from build123d import *

# Parameters (mm, degrees)
SKETCH1_R           = 18
BOSS_EXTRUDE1_DEPTH = 5
SKETCH2_R           = 18
SKETCH2_R_2         = 16.7
BOSS_EXTRUDE2_DEPTH = 25
SKETCH3_W           = 4
SKETCH3_H           = 4.625561496
CUT_EXTRUDE1_DEPTH  = 25


with BuildPart() as part:
    # Sketch1 → Boss-Extrude1 (new body)
    with BuildSketch(Plane(origin=(0, 0, 0), x_dir=(1, 0, 0), z_dir=(0, 1, 0))):
        with Locations(Location((0, 0, 0), (0, 0, 270))):
            Circle(SKETCH1_R)
    extrude(amount=BOSS_EXTRUDE1_DEPTH)

    # Sketch2 → Boss-Extrude2 (add)
    with BuildSketch(Plane(origin=(0, 5, 0), x_dir=(1, 0, 0), z_dir=(0, 1, 0))):
        with Locations(Location((0, 0, 0), (0, 0, 270))):
            Circle(SKETCH2_R)
        with Locations(Location((0, 0, 0), (0, 0, 270))):
            Circle(SKETCH2_R_2, mode=Mode.SUBTRACT)
    extrude(amount=BOSS_EXTRUDE2_DEPTH)

    # Sketch3 → Cut-Extrude1 (cut)
    with BuildSketch(Plane(origin=(0, 30, 0), x_dir=(1, 0, 0), z_dir=(0, 1, 0))):
        with Locations((0, 16.7)):
            Rectangle(SKETCH3_W, SKETCH3_H)
    extrude(amount=-CUT_EXTRUDE1_DEPTH, mode=Mode.SUBTRACT)

    # Cut-Loft1: read off the stored shape, not the designer's step
    # Cut-Loft1: loft between two sections, ruled curve by curve
    cut_loft1_from = [
        Edge.make_bspline([(-1.712462043, 0, -8.966813787), (-1.626363192, 0, -8.824108617), (-1.511615223, 0, -8.673150149), (-1.197727621, 0, -8.384153579), (-0.9972614, 0, -8.245981525), (-0.502854414, 0, -8.045966083), (-0.20751606, 0, -7.986207367), (0.419056865, 0, -8.019390239), (0.747775872, 0, -8.115340255), (1.318596553, 0, -8.459735659), (1.556747911, 0, -8.705797688), (1.878250858, 0, -9.244621024), (1.963090928, 0, -9.533754229), (2.016671796, 0, -10.064389259), (1.987908436, 0, -10.306155451), (1.878602966, 0, -10.718583333), (1.798560894, 0, -10.890481042), (1.626363192, 0, -11.175891383), (1.511615223, 0, -11.326849851), (1.197727621, 0, -11.615846421), (0.9972614, 0, -11.754018475), (0.502854414, 0, -11.954033917), (0.20751606, 0, -12.013792633), (-0.419056865, 0, -11.980609761), (-0.747775872, 0, -11.884659745), (-1.318596553, 0, -11.540264341), (-1.556747911, 0, -11.294202312), (-1.878250858, 0, -10.755378976), (-1.963090928, 0, -10.466245771), (-2.016671796, 0, -9.935610741), (-1.987908436, 0, -9.693844549), (-1.878602966, 0, -9.281416667), (-1.798560894, 0, -9.109518958), (-1.712462043, 0, -8.966813787)], [0, 0, 0, 0, 0.0625, 0.0625, 0.125, 0.125, 0.1875, 0.1875, 0.25, 0.25, 0.3125, 0.3125, 0.375, 0.375, 0.4375, 0.4375, 0.5, 0.5, 0.5625, 0.5625, 0.625, 0.625, 0.6875, 0.6875, 0.75, 0.75, 0.8125, 0.8125, 0.875, 0.875, 0.9375, 0.9375, 1, 1, 1, 1], 3),
    ]
    cut_loft1_to = [
        Edge.make_bspline([(-1.509327554, 5, -13.687776568), (-1.399975601, 5, -13.561999272), (-1.260982153, 5, -13.433017192), (-0.902081628, 5, -13.202290388), (-0.680844687, 5, -13.100641787), (-0.15941128, 5, -12.988607658), (0.14180355, 5, -12.980516047), (0.75334128, 5, -13.120930922), (1.06066884, 5, -13.271968541), (1.563778024, 5, -13.709376352), (1.756077925, 5, -13.9927195), (1.980154065, 5, -14.578795106), (2.014020397, 5, -14.8782094), (1.975571807, 5, -15.410155027), (1.905670109, 5, -15.643375898), (1.727083916, 5, -16.030869661), (1.618679506, 5, -16.186446136), (1.399975601, 5, -16.438000728), (1.260982153, 5, -16.566982808), (0.902081628, 5, -16.797709612), (0.680844687, 5, -16.899358213), (0.15941128, 5, -17.011392342), (-0.14180355, 5, -17.019483953), (-0.75334128, 5, -16.879069078), (-1.06066884, 5, -16.728031459), (-1.563778024, 5, -16.290623648), (-1.756077925, 5, -16.0072805), (-1.980154065, 5, -15.421204894), (-2.014020397, 5, -15.1217906), (-1.975571807, 5, -14.589844973), (-1.905670109, 5, -14.356624102), (-1.727083916, 5, -13.969130339), (-1.618679506, 5, -13.813553864), (-1.509327554, 5, -13.687776568)], [0, 0, 0, 0, 0.0625, 0.0625, 0.125, 0.125, 0.1875, 0.1875, 0.25, 0.25, 0.3125, 0.3125, 0.375, 0.375, 0.4375, 0.4375, 0.5, 0.5, 0.5625, 0.5625, 0.625, 0.625, 0.6875, 0.6875, 0.75, 0.75, 0.8125, 0.8125, 0.875, 0.875, 0.9375, 0.9375, 1, 1, 1, 1], 3),
    ]
    cut_loft1 = Solid(Shell([*[Face.make_surface_from_curves(cut_loft1_from[k], cut_loft1_to[k]) for k in range(1)], Face(Wire(cut_loft1_from)), Face(Wire(cut_loft1_to))]))
    add(cut_loft1, mode=Mode.SUBTRACT)


solid = part.part
Verification items for the finished model (mm, model axes). A direction names the side the tool comes from. Give positions to 0.01 mm unless a question says otherwise; leave off trailing zeros. Order: outer loops, then holes, each group sorted by start corner. A loop starts at its lowest first (then second) coordinate and runs counter-clockwise, first axis right, second up. Notation, with made-up numbers: M 31,-24.5 L 69,-24.5 A29 cw 69,10.5 Z; hole C -3.75,-31 d7. An arc over 180 degrees is marked long. Answer as a JSON object with one key per item and string values. Group by question number.
1) Depth check by flat-ended pin: pin 1 Ø5 at (x, z) = (11.5, 5) entering from +Y; pin 2 Ø1 at (y, z) = (14, -9) entering from -X; pin 3 Ø1 at (y, z) = (15, -17) entering from -X. Enter the tip coordinate at first touch or a pass-through.
2) Access from +Z, -Z, +X, -X, +Y, -Y to the whole of each face (thin tool, end or side, straight path). Record for faces 1 (the face through (2, 18, -17)), 2 (the face through (15, 30, 8)).
3) Mould release check, pull along X, two halves, no side actions. Record for faces 3 (the face through (5.407, 14.79, 17.169)), 4 (the face through (0, 5, -1)), 5 (the face through (0, 0, 0)): released by +X, released by -X, zero draft, split by the parting line, or undercut.
4) Cross-section at A-A (x = -4). Enter the section's corners in (y, z), then the cut area to 3 significant figures.
5) Cross-section at B-B (z = -6). Enter the section's corners in (x, y), then the cut area to 3 significant figures.
6) Scan lines: line 1 along Y through (x, z) = (10, 12.5); line 2 along Z through (x, y) = (-6, 17); line 3 along Z through (x, y) = (-7.5, 24). Record each from-to range of solid material in increasing order. Write a range as [from, to].
7) Cross-section at C-C (y = 26.5). Enter the section's corners in (x, z), then the cut area to 3 significant figures.
Result sheet:
{
 "1": {"pin 1": "stops at y = 5", "pin 2": "stops at x = -15.87", "pin 3": "stops at x = -7.19"},
 "2": {"face 1": "-Z, +Y", "face 2": "+Z, -Z, +X, -X, +Y"},
 "3": {"face 3": "split by the parting line", "face 4": "undercut", "face 5": "zero draft"},
 "4": {"outline": "M 0,-17.55 L 30,-17.55 L 30,-16.21 L 5,-16.21 L 5,16.21 L 30,16.21 L 30,17.55 L 0,17.55 Z", "area": "242 mm2"},
 "5": {"outline": "M -16.97,0 L 16.97,0 L 16.97,30 L 15.58,30 L 15.58,5 L -15.58,5 L -15.58,30 L -16.97,30 Z", "area": "239 mm2"},
 "6": {"line 1": "y = [0, 5]", "line 2": "z = [-16.97, -15.58], [15.58, 16.97]", "line 3": "z = [-16.36, -14.92], [14.92, 16.36]"},
 "7": {"outline": "M -2,-17.89 L -2,-16.58 A16.7 cw long 2,-16.58 L 2,-17.89 A18 ccw long Z", "area": "137 mm2"}
}
